Geometry: final body of the model. Coordinates: model frame, mm. A direction names the side the tool comes from. Round coordinates to 2 decimals unless told otherwise and drop trailing zeros. Write each loop counter-clockwise with the first axis right and the second up, starting at its lowest first coordinate (ties: lowest second). Pieces come first, ordered by that corner, then holes. Notation, with made-up numbers: M 0,20.25 L 16,20.25 A17 cw 16,29.25 Z; hole C -10.75,61 d5. An arc over 180 degrees is marked long. Use one line per item in the form item = value. Start each with the question number.
Item 1: Ray query, probe 1 along Z at (x, y) = (2, 6.5); probe 2 along Z at (x, y) = (0, 7); probe 3 along Z at (x, y) = (21.5, 44). Return the intervals inside material, ascending.
Item 2: Section query B-B (y = 28). Return loops of the section in (x, z) (3 decimals), and give its area (3 significant figures).
Item 3: Reachability of faces 1 (the flat face through (19.14, 25.04, -4.74)), 2 (the cylindrical face through (2.902, 4.837, -1.252)), 3 (the flat face through (0, 16.51, -3)) from +Z, -Z, +X, -X, +Y, -Y: full face, straight path, thin tool, end or side. Return the list, or none.
Item 4: Pin query (flat end, axial travel): pin 1 Ø3 at (x, y) = (-3.5, 32) entering from +Z; pin 2 Ø1 at (x, y) = (-5, 40) entering from -Z; pin 3 Ø1.5 at (x, y) = (-6.5, 32.5) entering from -Z; pin 4 Ø1.5 at (x, y) = (7, 9.5) entering from +Z. Return the tip coordinate at first contact, or that it passes through.
Item 5: Pull-direction query (Z, two-part tool) for faces 4 (the flat face through (6, 50.8, -3)), 5 (the flat face through (2, 8, -3.81)), 6 (the cylindrical face through (-1.586, 8.139, -3.236)), 7 (the flat face through (6, 25, -6.35)); classes: pulls with the +Z half, pulls with the -Z half, needs draft (parallel to the pull), parting line crosses it, or undercut.
Item 6: Section query C-C (x = 19.5). Return loops of the section in (y, z).
from build123d import *

# Parameters (mm, degrees)
BOSS_EXTRUDE1_DEPTH = 50.8
CUT_EXTRUDE1_DEPTH  = 16.51
SKETCH3_R           = 0.635
CUT_EXTRUDE2_DEPTH  = 3.175


with BuildPart() as part:
    # Sketch1 → Boss-Extrude1 (new body)
    with BuildSketch(Plane(origin=(0, 0, 0), x_dir=(1, 0, 0), z_dir=(0, 1, 0))):
        Polygon((0, 6.35), (-12.7, 3.1623), (0, 0), (12.7, 0), (25.4, 3.175), (12.7, 6.35), align=None)
    extrude(amount=BOSS_EXTRUDE1_DEPTH)

    # Sketch2 → Cut-Extrude1 (cut)
    with BuildSketch(Plane.XZ):
        with BuildLine():
            Line((3.175, -2.54), (3.175, -3.81))
            Line((3.175, -3.81), (1.454967783, -3.81))
            ThreePointArc((1.454967783, -3.81), (-1.5875, -3.175), (1.454967783, -2.54))
            Line((1.454967783, -2.54), (3.175, -2.54))
        make_face()
    extrude(amount=-CUT_EXTRUDE1_DEPTH, mode=Mode.SUBTRACT)

    # Sketch3 → Cut-Extrude2 (cut)
    with BuildSketch(Plane.XY):
        with Locations((2.31521, 5.08)):
            Circle(SKETCH3_R)
        with Locations((2.31521, 10.16)):
            Circle(SKETCH3_R)
    extrude(amount=-CUT_EXTRUDE2_DEPTH, mode=Mode.SUBTRACT)


solid = part.part
Working result:
q1.probe_1 = -6.35 to -3.81, -2.54 to 0
q1.probe_2 = -6.35 to -4.76, -1.59 to 0
q1.probe_3 = -4.15 to -2.2
q2.outline = M -12.7,-3.162 L 0,-6.35 L 12.7,-6.35 L 25.4,-3.175 L 12.7,0 L 0,0 Z
q2.area = 161 mm²
q3.face_1 = -Z, +X, +Y, -Y
q3.face_2 = +Z
q3.face_3 = -Y
q4.pin_1 = -0.5
q4.pin_2 = -5.22
q4.pin_3 = -4.91
q4.pin_4 = 0
q5.face_4 = needs draft
q5.face_5 = undercut
q5.face_6 = undercut
q5.face_7 = pulls with the -Z half
q6.outline = M 0,-4.65 L 50.8,-4.65 L 50.8,-1.7 L 0,-1.7 Z
